Could you check a few things on this model? Use its own coordinates, in mm. Face numbers are marked on the shaded views. A direction names the side the tool comes from. Give positions to 0.01 mm unless a question says otherwise; leave off trailing zeros. Order: outer loops, then holes, each group sorted by start corner. A loop starts at its lowest first (then second) coordinate and runs counter-clockwise, first axis right, second up. Notation, with made-up numbers: (63.25, 84) -> (84.25, 84) arc R16 ccw to (84.25, 115) -> close; hole circle Ø9 at (63, 37.5). An arc over 180 degrees is marked (long way). Write each question's results on one line, items separated by ' | '.
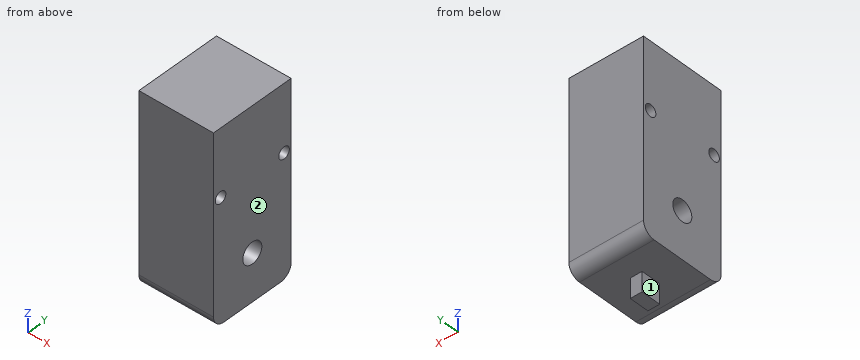
Autodesk Fusion 360 part; units mm, degrees
sketch "Case base" plane through (0, 0, 0) normal (1, 0, 0) x (0, 1, 0)
  line L0 (-11, 24) -> (11, 24)
  line L1 (11, 24) -> (11, -21)
  line L2 (8, -24) -> (-8, -24)
  line L3 (-11, -21) -> (-11, 24)
  line L4 (-11, 24) -> (11, -24) construction
  line L5 (11, 24) -> (-11, -24) construction
  arc A0 (-11, -21) -> (-8, -24) centre (-8, -21) ccw
  arc A1 (8, -24) -> (11, -21) centre (8, -21) ccw
  dimension "d5" = 22
  dimension "d6" = 48
  dimension "d7" = 3
  dimension "d8" = 3
extrude "Case width" add sketch "Case base" along normal blind 19
sketch "Pin base" plane through (0, 0, -24) normal (0, 0, -1) x (1, 0, 0)
  line L0 (0, 8) -> (0, -8)
  line L1 (0, -8) -> (19, -8)
  line L2 (19, -8) -> (19, 8)
  line L3 (19, 8) -> (0, 8)
  line L4 (0, 0) -> (19, 0) construction
  line L5 (11, 2.5) -> (8, 2.5)
  line L6 (8, 2.5) -> (8, -2.5)
  line L7 (8, -2.5) -> (11, -2.5)
  line L8 (11, -2.5) -> (11, 2.5)
  line L9 (11, 2.5) -> (8, -2.5) construction
  line L10 (8, 2.5) -> (11, -2.5) construction
  point P0 (9.5, 0)
  dimension "d11" = 5
  dimension "d12" = 3
extrude "Pin base (1)" add sketch "Pin base" along normal blind 5 contours L5 L6 L7 L8
sketch "Pin hole" plane through (11, 0, 0) normal (1, 0, 0) x (0, 1, 0)
  line L0 (2.5, -24) -> (-2.5, -24)
  line L1 (-2.5, -24) -> (-2.5, -29)
  line L2 (-2.5, -29) -> (2.5, -29)
  line L3 (2.5, -29) -> (2.5, -24)
  circle A0 centre (0, -26.5) radius 1.5
  dimension "d15" = 3
extrude "Pin hole (1)" cut sketch "Pin hole" along normal through all contours A0
sketch "Case axis" plane through (19, 0, 0) normal (1, 0, 0) x (0, 1, 0)
  arc A0 (-11, -21) -> (-8, -24) centre (-8, -21) ccw
  line L0 (-8, -24) -> (8, -24)
  arc A1 (8, -24) -> (11, -21) centre (8, -21) ccw
  line L1 (11, -21) -> (11, 24)
  line L2 (11, 24) -> (-11, 24)
  line L3 (-11, 24) -> (-11, -21)
  line L4 (0, -24) -> (0, -12) construction
  circle A2 centre (0, -12) radius 2.7
  dimension "d17" = 12
  dimension "d18" = 5.4
extrude "Case axis (1)" cut sketch "Case axis" against normal through all contours A2
sketch "Case hole" plane through (19, 0, 0) normal (1, 0, 0) x (0, 1, 0)
  circle A0 centre (0, -12) radius 2.7
  arc A1 (-11, -21) -> (-8, -24) centre (-8, -21) ccw
  line L0 (-8, -24) -> (8, -24)
  arc A2 (8, -24) -> (11, -21) centre (8, -21) ccw
  line L1 (11, -21) -> (11, 24)
  line L2 (11, 24) -> (-11, 24)
  line L3 (-11, 24) -> (-11, -21)
  line L4 (-11, 22) -> (-9, 22) construction
  line L5 (-9, 24) -> (-9, 7) construction
  circle A3 centre (-9, 7) radius 1.5
  dimension "d20" = 2
  dimension "d21" = 17
  dimension "d22" = 3
extrude "Case hole (1)" cut sketch "Case hole" against normal through all contours A3
mirror "Case holes" about plane through (0, 0, 0) normal (0, 1, 0) of "Case hole (1)"
Q1. Suppose I cut it at A-A on z = 7. Please give me the cut outline in (x, y).
Here are the results:
outline: (0, -11) -> (19, -11) -> (19, -10.5) -> (0, -10.5) -> close; (0, -7.5) -> (19, -7.5) -> (19, 7.5) -> (0, 7.5) -> close; (0, 10.5) -> (19, 10.5) -> (19, 11) -> (0, 11) -> close
Q2. I'm going to push flat-ended pins straight in: pin 1 Ø4.5 at (y, z) = (0, -12) entering from -X; pin 2 Ø5 at (x, y) = (8.5, -8) entering from -Z; pin 3 Ø2.5 at (x, z) = (10, -26.5) entering from -Y; pin 4 Ø2.5 at (y, z) = (-0.5, -25.5) entering from +X. Where does each tip first touch, or does it pass through?
Here are the results:
pin 1: passes through | pin 2: stops at z = -24 | pin 3: stops at y = -2.5 | pin 4: stops at x = 11
Q3. I need wall thicknesses on line 1 along Z through (x, y) = (5.25, 0); line 2 along Y through (x, z) = (2, -11); line 3 along Z through (x, y) = (10.75, 9). Which ranges of each line are inside material? Lowest first, please.
Here are the results:
line 1: z = -24 to -14.7, -9.3 to 24 | line 2: y = -11 to -2.51, 2.51 to 11 | line 3: z = -23.83 to 5.5, 8.5 to 24
Q4. Suppose I cut it at C-C on y = 0. Please give me the cut outline in (x, z), and give its area (3 significant figures).
Here are the results:
outline: (0, -24) -> (8, -24) -> (8, -29) -> (11, -29) -> (11, -24) -> (19, -24) -> (19, -14.7) -> (0, -14.7) -> close; (0, -9.3) -> (19, -9.3) -> (19, 24) -> (0, 24) -> close | area: 824 mm²
Q5. Suppose I cut it at D-D on y = -9. Please give me the cut outline in (x, z), and give its area (3 significant figures).
Here are the results:
outline: (0, -23.83) -> (19, -23.83) -> (19, 5.5) -> (0, 5.5) -> close; (0, 8.5) -> (19, 8.5) -> (19, 24) -> (0, 24) -> close | area: 852 mm²
Q6. Suppose I cut it at B-B on x = 8.75. Please give me the cut outline in (y, z).
Here are the results:
outline: (-11, -21) arc R3 ccw to (-8, -24) -> (-2.5, -24) -> (-2.5, -29) -> (2.5, -29) -> (2.5, -24) -> (8, -24) arc R3 ccw to (11, -21) -> (11, 24) -> (-11, 24) -> close; hole circle Ø3 at (-9, 7); hole circle Ø5.4 at (0, -12); hole circle Ø3 at (9, 7)
Q7. For the marked faces 1 and 2, which set-ups out of +Z, -Z, +X, -X, +Y, -Y let a thin tool reach every point of the face, with its end or its side?
Here are the results:
face 1: -Z, -X, +Y, -Y | face 2: +Z, -Z, +X, +Y, -Y
